from build123d import *

# Parameters (mm, degrees)
F0_R      = 7.5
F1_DEPTH  = 10
F4_R      = 5
F5_DEPTH  = 18
F6_R      = 1
F7_DEPTH  = 25.8740546369
F10_R     = 6
F10_R_2   = 5
F11_DEPTH = 1.5


# Not quite as in the source:
# - a fillet or chamfer that OpenCascade refuses, or shapes differently, is made with other operations: its cross-section is extruded or revolved along the edge and cut away or added


with BuildPart() as f1:
    # F0 (on Top) → F1 (new body)
    with BuildSketch(Plane.XY):
        Circle(F0_R)
    extrude(amount=F1_DEPTH)

    # F2 (on Front) → F3 (revolve, cut)
    with BuildSketch(Plane.XZ):
        with BuildLine():
            Line((10, 10), (0, 10))
            Line((0, 10), (0, 6))
            ThreePointArc((0, 6), (5.4685094621, 6.8287263446), (10, 10))
        make_face()
    revolve(axis=Axis((0, 0, 8), (0, 0, -1)), mode=Mode.SUBTRACT)

    # F4 (on face) → F5 (join)
    with BuildSketch(Plane(origin=(0, 0, 0), x_dir=(1, 0, 0), z_dir=(0, 0, -1))):
        Circle(F4_R)
    extrude(amount=F5_DEPTH)

    # F6 (on face) → F7 (cut, through all)
    with BuildSketch(Plane(origin=(0, 0, -18), x_dir=(1, 0, 0), z_dir=(0, 0, -1))):
        Circle(F6_R)
    extrude(amount=-F7_DEPTH, mode=Mode.SUBTRACT)

    # F8: chamfer of 4.5 on 1 edges, made by hand

    # F8_s1 → F8_t2 (revolve, cut)
    with BuildSketch(Plane.XZ):
        Polygon((5, -13.5), (0.5, -18), (5, -18), align=None)
    revolve(axis=Axis((0, 0, -18), (0, 0, -1)), mode=Mode.SUBTRACT)

    # F10 (on offset) → F11 (join)
    with BuildSketch(Plane.XY.offset(-10)):
        Circle(F10_R)
        Circle(F10_R_2, mode=Mode.SUBTRACT)
    extrude(amount=-F11_DEPTH)


solid = f1.part
Could you check a few things on this model? Use its own coordinates, in mm. A direction names the side the tool comes from. Coordinates: 2 decimals unless noted, no trailing zeros. Order: outer loops, then holes, each group sorted by start corner. A loop starts at its lowest first (then second) coordinate and runs counter-clockwise, first axis right, second up. Notation, with made-up numbers: (32.25, 57) -> (45.25, 57) arc R31 ccw to (45.25, 86) -> close; hole circle Ø7 at (-0.5, 88). An arc over 180 degrees is marked (long way). One line per item, written item: value. Start each with the question number.
1) Imagine slicing it at B-B on z = -13. List the corners of the cut face in (x, y) for me.
2) If I drill on L1, parallel to X at y = 0, z = 1; L2, parallel to X at y = 0, z = -4.5, over which ranges is the centre line in solid material (lowest first)? Write a range as [from, to].
3) Imagine slicing it at A-A on z = 2.75. List the corners of the cut face in (x, y) for me, plus the area to 3 significant figures.
4) Which directions (+Z, -Z, +X, -X, +Y, -Y) give clear straight access to the entire face, cutting with the end or side of a thin tool? Please do faces 4 (the cylindrical face through (-1.08, 4.88, -12.49)), 5 (the cylindrical face through (-7.493, 0.33, 3.881)), 6 (the flat face through (-4, 4, -10)).
5) We'd pull the mould along Z, two halves only. Please class faces 1 (the cylindrical face through (-1.08, 4.88, -4.93)), 2 (the flat face through (-4, 4, -11.5)), 3 (the cylindrical face through (0, 1, -6)): +Z half, -Z half, draft (parallel to the pull), parting line (faces both ways), or undercut.
6) I'm going to push flat-ended pins straight in: pin 1 (3 mm diameter, centred on x = -4.5, z = 0, fed in from +Y); pin 2 (4 mm diameter, centred on x = 1, y = -4, fed in from +Z); pin 3 (2 mm diameter, centred on x = 2.5, y = -6, fed in from -Z). Where does each tip first touch, or does it pass through?
Answer list:
1. outline: circle Ø10 at (0, 0); hole circle Ø2 at (0, 0)
2. L1: x = [-7.5, -1], [1, 7.5]
2. L2: x = [-5, -1], [1, 5]
3. outline: circle Ø15 at (0, 0); hole circle Ø2 at (0, 0)
3. area: 174 mm2
4. face 4: -Z
4. face 5: +Z, -Z
4. face 6: none
5. face 1: undercut
5. face 2: -Z half
5. face 3: draft
6. pin 1: stops at y = 6.87
6. pin 2: stops at z = 7.11
6. pin 3: stops at z = -11.5
